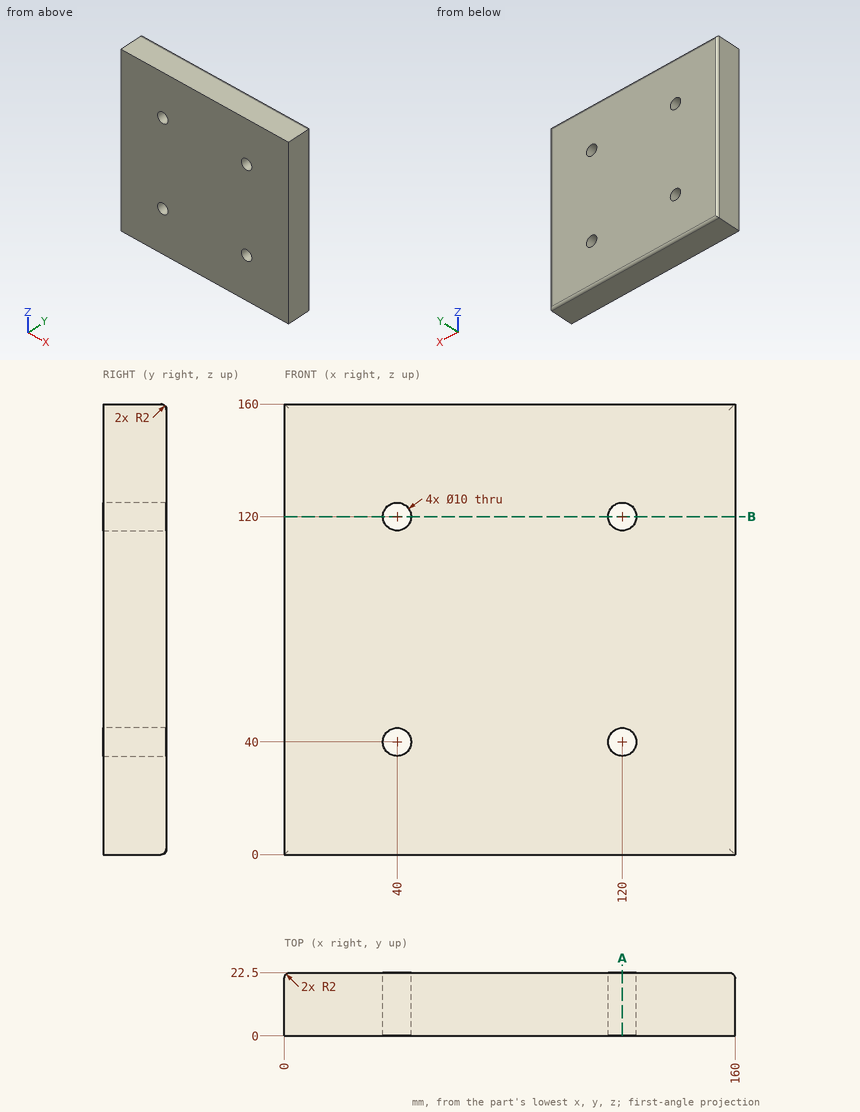
Drawing for the job (mm, zero at the part's lowest x, y, z). Give positions to 0.01 mm unless a question says otherwise; leave off trailing zeros. Write each loop counter-clockwise with the first axis right and the second up, starting at its lowest first coordinate (ties: lowest second). Pieces come first, ordered by that corner, then holes. Notation, with made-up numbers: (14.25, 87) -> (49.25, 87) arc R7 ccw to (49.25, 96) -> close; hole circle Ø5 at (-16, 70.5). An arc over 180 degrees is marked (long way). Put each result on its own line as item: value. Start each with the question number.
Item 1: Pin check, flat tip, straight feed: pin 1 Ø9 at (x, z) = (40, 120) entering from -Y. Stop position of the tip, or through.
Item 2: Cut at A-A (x = 120). List the corners of the cut face in (y, z).
Item 3: Cut at B-B (z = 120). List the corners of the cut face in (x, y), then the cut area to 3 significant figures.
Item 4: Wall check: L1, parallel to X at y = 11, z = 40. Give the ranges that are in metal, low to high. Write a range as [from, to].
Answer list:
1. pin 1: passes through
2. outline: (0, 0) -> (20.5, 0) arc R2 ccw to (22.5, 2) -> (22.5, 35) -> (0, 35) -> close; (0, 45) -> (22.5, 45) -> (22.5, 115) -> (0, 115) -> close; (0, 125) -> (22.5, 125) -> (22.5, 158) arc R2 ccw to (20.5, 160) -> (0, 160) -> close
3. outline: (0, 0) -> (35, 0) -> (35, 22.5) -> (2, 22.5) arc R2 ccw to (0, 20.5) -> close; (45, 0) -> (115, 0) -> (115, 22.5) -> (45, 22.5) -> close; (125, 0) -> (160, 0) -> (160, 20.5) arc R2 ccw to (158, 22.5) -> (125, 22.5) -> close
3. area: 3,150 mm2
4. L1: x = [0, 35], [45, 115], [125, 160]
